from build123d import *

# Parameters (mm, degrees)
SKETCH1_W               = 60
SKETCH1_H               = 40
BOSS_EXTRUDE1_DEPTH     = 15
SKETCH3_R               = 5.2
CUT_EXTRUDE1_DEPTH      = 63
SKETCH4_W               = 7
SKETCH4_H               = 40
BOSS_EXTRUDE2_DEPTH     = 30
SKETCH5_R               = 5
CUT_EXTRUDE2_DEPTH      = 5
SKETCH6_R               = 5
CUT_EXTRUDE3_DEPTH      = 4
SKETCH7_R               = 2.5
CUT_EXTRUDE4_DEPTH      = 42
SKETCH8_R               = 15.75
CUT_EXTRUDE5_DEPTH      = 2.5
SKETCH9_R               = 1.5
CUT_EXTRUDE6_DEPTH      = 54
CUT_EXTRUDE6_DEPTH_BACK = 8


with BuildPart() as part:
    # Sketch1 → Boss-Extrude1 (new body)
    with BuildSketch(Plane.XY):
        with Locations((12.222222222, 0.91503268)):
            Rectangle(SKETCH1_W, SKETCH1_H)
    extrude(amount=BOSS_EXTRUDE1_DEPTH)

    # Sketch3 → Cut-Extrude1 (cut)
    with BuildSketch(Plane(origin=(42.222222222, 0, 0), x_dir=(0, 0, -1), z_dir=(1, 0, 0))):
        with Locations((-3, -11.48496732)):
            Circle(SKETCH3_R)
        with Locations((-3, 13.31503268)):
            Circle(SKETCH3_R)
    extrude(amount=-CUT_EXTRUDE1_DEPTH, mode=Mode.SUBTRACT)

    # Sketch4 → Boss-Extrude2 (add)
    with BuildSketch(Plane.XY.offset(15)):
        with Locations((38.722222222, 0.91503268)):
            Rectangle(SKETCH4_W, SKETCH4_H)
    boss_extrude2 = extrude(amount=BOSS_EXTRUDE2_DEPTH)

    # Sketch5 → Cut-Extrude2 (cut)
    with BuildSketch(Plane(origin=(42.222222222, 0, 0), x_dir=(0, 0, -1), z_dir=(1, 0, 0))):
        with Locations((-26, 0.91503268)):
            Circle(SKETCH5_R)
    cut_extrude2 = extrude(amount=-CUT_EXTRUDE2_DEPTH, mode=Mode.SUBTRACT)

    # Mirror1: Boss-Extrude2, Cut-Extrude2 across plane
    add(boss_extrude2.mirror(Plane.ZY.offset(-12.222222222)))
    add(cut_extrude2.mirror(Plane.ZY.offset(-12.222222222)), mode=Mode.SUBTRACT)

    # Sketch6 → Cut-Extrude3 (cut)
    with BuildSketch(Plane(origin=(0, 0, 0), x_dir=(-1, 0, 0), z_dir=(0, 0, -1))):
        with Locations((-12.222222222, 0.91503268)):
            Circle(SKETCH6_R)
    extrude(amount=-CUT_EXTRUDE3_DEPTH, mode=Mode.SUBTRACT)

    # Sketch7 → Cut-Extrude4 (cut, through all)
    with BuildSketch(Plane(origin=(0, 0, 4), x_dir=(-1, 0, 0), z_dir=(0, 0, -1))):
        with Locations((-12.222222222, 0.91503268)):
            Circle(SKETCH7_R)
    extrude(amount=-CUT_EXTRUDE4_DEPTH, mode=Mode.SUBTRACT)

    # Sketch8 → Cut-Extrude5 (cut)
    with BuildSketch(Plane.XY.offset(15)):
        with Locations((12.222222222, 0.91503268)):
            Circle(SKETCH8_R)
    extrude(amount=-CUT_EXTRUDE5_DEPTH, mode=Mode.SUBTRACT)

    # Sketch9 → Cut-Extrude6 (cut, two sides)
    with BuildSketch(Plane.ZY.offset(-35.222222222)) as cut_extrude6_sk:
        with Locations((26, 0.91503268)):
            Circle(SKETCH9_R)
    extrude(amount=CUT_EXTRUDE6_DEPTH, mode=Mode.SUBTRACT)
    extrude(cut_extrude6_sk.sketch, amount=-CUT_EXTRUDE6_DEPTH_BACK, mode=Mode.SUBTRACT)


solid = part.part
Input: part model. Units: mm. Frame: model coordinates. A direction names the side the tool comes from. Coordinates: 2 decimals unless noted, no trailing zeros. Loops run counter-clockwise (first coordinate to the right, second up) from the corner with the lowest first, then second, coordinate; pieces in that order, holes last. Notation, with made-up numbers: (-19.5, 26.25) -> (4.5, 26.25) arc R12 ccw to (4.5, 39.25) -> close; hole circle Ø2 at (11.5, 88). An arc over 180 degrees is marked (long way). Write item = value, one per line. Start each with the question number.
Item 1: Cut plane A-A, the plane z = 26. Return loops of the section in (x, y), plus the area to 3 significant figures.
Item 2: Reachability of faces 5 (the face through (16, 1, 12.5)), 6 (the face through (35.222, 1, 30)), 7 (the face through (37.222, 2.1, 27.2)) from +Z, -Z, +X, -X, +Y, -Y: full face, straight path, thin tool, end or side. Return the list, or none.
Item 3: Cut plane B-B, the plane z = 40. Return loops of the section in (x, y), plus the area to 3 significant figures.
Item 4: Cut plane C-C, the plane z = 3. Return loops of the section in (x, y).
Item 5: First-contact query: P1, Ø8, axis at y = 0.5, z = 26.5, coming from the -X side; P2, Ø1.5, axis at x = 4, y = 14, coming from the +Z side; P3, Ø6, axis at x = 12.22, y = 0.92, coming from the -Z side. Flat tips, straight axial feed; report the tip coordinate or a pass-through.
Item 6: Mould query, pull axis Z, two halves, no side actions, for faces 1 (the face through (36.21, 0.98, 24.5)), 2 (the face through (-15, 1, 31)), 3 (the face through (15, 0, 4)), 4 (the face through (26.77, -5.12, 13.77)). Classes: pulls with the +Z half, pulls with the -Z half, needs draft (parallel to the pull), parting line crosses it, or undercut.
Item 7: Cut plane D-D, the plane x = 13. Return loops of the section in (y, z), plus the area to 3 significant figures.
Item 8: Material intervals for line 1 (X direction, y = 5, z = 34); line 2 (Z direction, x = -13.5, y = 1); line 3 (Y direction, x = 14.5, z = 3), sorted ascending.
Ans:
q1.outline = (-17.78, -19.08) -> (-10.78, -19.08) -> (-10.78, -0.58) -> (-12.78, -0.58) -> (-12.78, -4.08) -> (-17.78, -4.08) -> close; (-17.78, 5.92) -> (-12.78, 5.92) -> (-12.78, 2.42) -> (-10.78, 2.42) -> (-10.78, 20.92) -> (-17.78, 20.92) -> close; (35.22, -19.08) -> (42.22, -19.08) -> (42.22, -4.08) -> (37.22, -4.08) -> (37.22, -0.58) -> (35.22, -0.58) -> close; (35.22, 2.42) -> (37.22, 2.42) -> (37.22, 5.92) -> (42.22, 5.92) -> (42.22, 20.92) -> (35.22, 20.92) -> close
q1.area = 448 mm²
q2.face_5 = +Z
q2.face_6 = +Z, +Y, -Y
q2.face_7 = +X
q3.outline = (-17.78, -19.08) -> (-10.78, -19.08) -> (-10.78, 20.92) -> (-17.78, 20.92) -> close; (35.22, -19.08) -> (42.22, -19.08) -> (42.22, 20.92) -> (35.22, 20.92) -> close
q3.area = 560 mm²
q4.outline = (-17.78, -19.08) -> (42.22, -19.08) -> (42.22, -16.68) -> (-17.78, -16.68) -> close; (-17.78, -6.28) -> (42.22, -6.28) -> (42.22, 8.12) -> (-17.78, 8.12) -> close; (-17.78, 18.52) -> (42.22, 18.52) -> (42.22, 20.92) -> (-17.78, 20.92) -> close; hole circle Ø10 at (12.22, 0.92)
q5.P1 = -12.78
q5.P2 = 15
q5.P3 = 4
q6.face_1 = undercut
q6.face_2 = undercut
q6.face_3 = pulls with the -Z half
q6.face_4 = needs draft
q7.outline = (-19.08, 0) -> (-15.73, 0) arc R5.2 cw (long way) to (-7.24, 0) -> (-4.02, 0) -> (-4.02, 4) -> (-1.46, 4) -> (-1.46, 12.5) -> (-14.82, 12.5) -> (-14.82, 15) -> (-19.08, 15) -> close; (3.29, 4) -> (5.85, 4) -> (5.85, 0) -> (9.07, 0) arc R5.2 cw (long way) to (17.56, 0) -> (20.92, 0) -> (20.92, 15) -> (16.65, 15) -> (16.65, 12.5) -> (3.29, 12.5) -> close
q7.area = 298 mm²
q8.line_1 = -17.78 to -10.78, 35.22 to 42.22
q8.line_2 = 0 to 21, 31 to 45
q8.line_3 = -19.08 to -16.68, -6.28 to -3.54, 5.37 to 8.12, 18.52 to 20.92
